```python
from build123d import *

# Parameters (mm, degrees)
SKETCH1_R               = 9.525
SKETCH1_R_2             = 2.599995
BOSS_EXTRUDE1_DEPTH     = 5
SKETCH2_R               = 25.4
BOSS_EXTRUDE2_DEPTH     = 0.75
SKETCH6_R               = 0.79375
CUT_EXTRUDE2_DEPTH      = 2.54
CUT_EXTRUDE3_REACH      = 45.566
CUT_EXTRUDE3_END_RADIUS = 2.599995
SKETCH7_R               = 1.4


with BuildPart() as part:
    # Sketch1 → Boss-Extrude1 (new body)
    with BuildSketch(Plane.XY):
        Circle(SKETCH1_R)
        Circle(SKETCH1_R_2, mode=Mode.SUBTRACT)
    extrude(amount=BOSS_EXTRUDE1_DEPTH)

    # Sketch2 → Boss-Extrude2 (add)
    with BuildSketch(Plane.XY.offset(5)):
        Circle(SKETCH2_R)
    extrude(amount=BOSS_EXTRUDE2_DEPTH)

    # Sketch6 → Cut-Extrude2 (cut)
    with BuildSketch(Plane.XY.offset(5.75)):
        Circle(SKETCH6_R)
    extrude(amount=-CUT_EXTRUDE2_DEPTH, mode=Mode.SUBTRACT)

    # Cut-Extrude3: up to this cylinder (the profile starts outside it)
    cut_extrude3_end = Plane(origin=(0, 0, 2.5), z_dir=(0, 0, -1)) * Cylinder(CUT_EXTRUDE3_END_RADIUS, 97.33199, mode=Mode.PRIVATE)
    # Sketch7 → Cut-Extrude3 (cut, up to the surface)
    with BuildSketch(Plane(origin=(0, 9.525, 0), x_dir=(1, 0, 0), z_dir=(0, 1, 0)), mode=Mode.PRIVATE) as cut_extrude3_sk1:
        with Locations(Location((0, -2.5, 0), (0, 0, 270))):
            Circle(SKETCH7_R)
    cut_extrude3_tool1 = extrude(cut_extrude3_sk1.sketch, amount=-CUT_EXTRUDE3_REACH, mode=Mode.PRIVATE) - cut_extrude3_end
    add(cut_extrude3_tool1.solids().sort_by_distance((0, 9.525, 2.5))[0], mode=Mode.SUBTRACT)


solid = part.part
```
CAD build for the part. Positions are in the model's coordinates, mm. A direction names the side the tool comes from. Round coordinates to 2 decimals unless told otherwise and drop trailing zeros. Order: outer loops, then holes, each group sorted by start corner. A loop starts at its lowest first (then second) coordinate and runs counter-clockwise, first axis right, second up. Notation, with made-up numbers: (35.25, 48.25) - (75.25, 48.25) arc R19 ccw to (75.25, 81.25) - close; hole circle Ø8 at (11.25, 34.5). An arc over 180 degrees is marked (long way). Use CSV: the item, a comma, the result in double quotes. Start each with the question number.
1) Tool access for faces 1 (the cylindrical face through (0.421, 5.909, 3.835)), 2 (the flat face through (2, -2, 0)), 3 (the flat face through (11, 0, 5)): list every direction of +Z, -Z, +X, -X, +Y, -Y with a clear straight run to the whole face (end or side of a thin tool).
2) Wall check: L1, parallel to Y at x = 0, z = 4.65 (3 decimals); L2, parallel to Y at x = 0, z = 5.55; L3, parallel to Z at x = 0, y = 15.5. Give the ranges that are in metal, low to high. Write a range as [from, to].
3) Saw through at A-A (x = 0). List the corners of the cut face in (y, z) (3 decimals), and give its area (3 significant figures).
4) Saw through at D-D (z = 2.5). List the corners of the cut face in (x, y) (3 decimals).
5) Saw through at C-C (x = -18). List the corners of the cut face in (y, z), and give its area (3 significant figures).
6) Two-plate mould, pull along X, no slides. Class faces 4 (the flat face through (5, 0, 5.75)), 5 (the cylindrical face through (-0.172, -0.775, 5.38)), 6 (the cylindrical face through (-5.506, -24.796, 5.37)): pulls with the +X half, pulls with the -X half, needs draft (parallel to the pull), parting line crosses it, or undercut.
7) Pin check, flat tips, straight feed: pin 1 Ø1.3 at (x, y) = (0, 0) entering from -Z (1 decimal); pin 2 Ø5 at (x, y) = (2, 17.5) entering from -Z; pin 3 Ø3 at (y, z) = (-8, 4.5) entering from -X. Stop position of each tip, or through.
8) Saw through at B-B (y = 0). List the corners of the cut face in (x, z) (3 decimals), and give its area (3 significant figures).
Values follow:
1,face 1,"+Y"
1,face 2,"-Z, +X, -X, +Y, -Y"
1,face 3,"-Z"
2,L1,"y = [-9.525, -2.6], [2.6, 9.525]"
2,L2,"y = [-25.4, -0.79], [0.79, 25.4]"
2,L3,"z = [5, 5.75]"
3,outline,"(-25.4, 5) - (-9.525, 5) - (-9.525, 0) - (-2.6, 0) - (-2.6, 5) - (-0.794, 5) - (-0.794, 5.75) - (-25.4, 5.75) - close; (0.794, 5) - (2.6, 5) - (2.6, 3.9) - (9.525, 3.9) - (9.525, 5) - (25.4, 5) - (25.4, 5.75) - (0.794, 5.75) - close; (2.6, 0) - (9.525, 0) - (9.525, 1.1) - (2.6, 1.1) - close"
3,area,"86.8 mm2"
4,outline,"(-1.4, 2.191) - (-1.4, 9.422) arc R9.525 ccw (long way) to (1.4, 9.422) - (1.4, 2.191) arc R2.6 cw (long way) to start"
5,outline,"(-17.92, 5) - (17.92, 5) - (17.92, 5.75) - (-17.92, 5.75) - close"
5,area,"26.9 mm2"
6,face 4,"needs draft"
6,face 5,"undercut"
6,face 6,"parting line crosses it"
7,pin 1,"passes through"
7,pin 2,"stops at z = 5"
7,pin 3,"stops at x = -24.53"
8,outline,"(-25.4, 5) - (-9.525, 5) - (-9.525, 0) - (-2.6, 0) - (-2.6, 5) - (-0.794, 5) - (-0.794, 5.75) - (-25.4, 5.75) - close; (0.794, 5) - (2.6, 5) - (2.6, 0) - (9.525, 0) - (9.525, 5) - (25.4, 5) - (25.4, 5.75) - (0.794, 5.75) - close"
8,area,"106 mm2"
